Source: three-view drawing plus pictorial views. Frame: mm from the lowest corner of the part. Give positions to 0.01 mm unless a question says otherwise; leave off trailing zeros. Loops run counter-clockwise (first coordinate to the right, second up) from the corner with the lowest first, then second, coordinate; pieces in that order, holes last. Notation, with made-up numbers: (3.5, 64) -> (47.5, 64) arc R25 ccw to (47.5, 81) -> close; hole circle Ø2 at (-1.5, 67.25). An arc over 180 degrees is marked (long way). Answer as a JSON object with one key per item and string values. Group by question number.
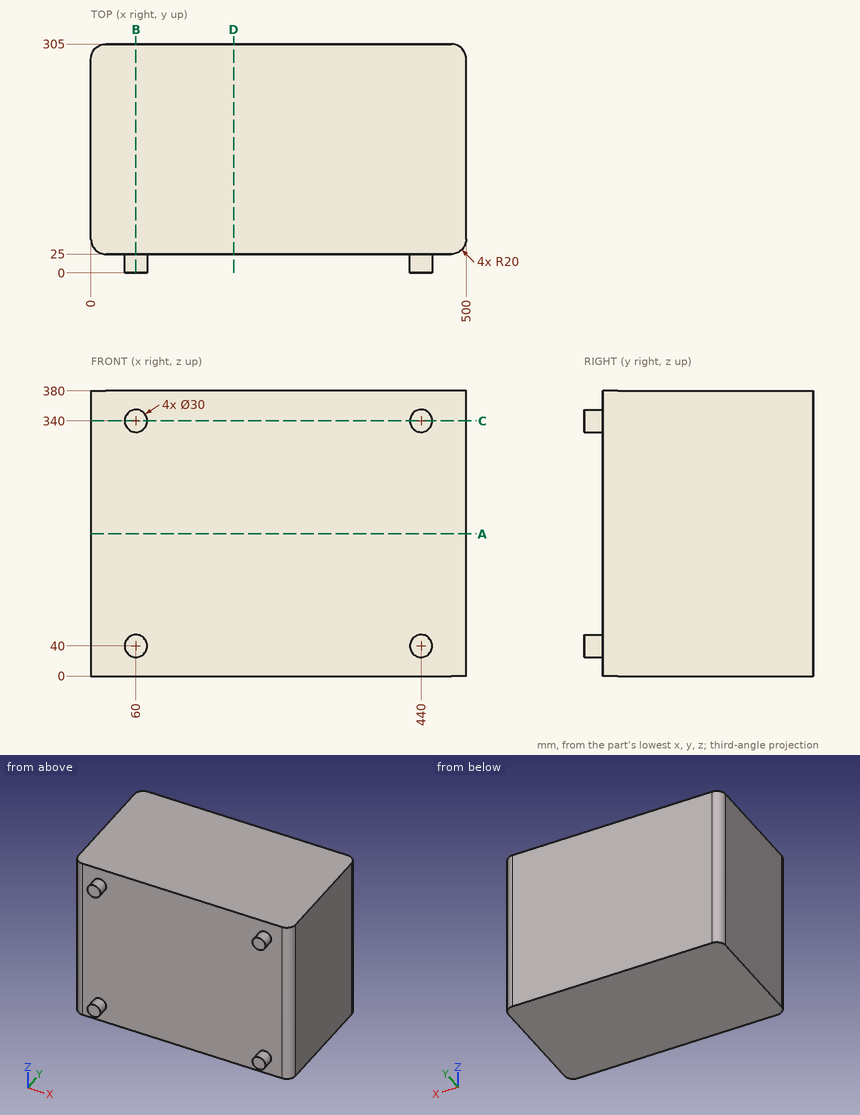
Q1. Section B-B on x = 60. Return the cut outline in (y, z), then the cut area to 3 significant figures.
Q2. Pin query (flat end, axial travel): pin 1 Ø1.5 at (x, y) = (120.5, 48.5) entering from -Z. Return the tip coordinate at first contact, or that it passes through.
Q3. Section A-A on z = 189.5. Return the cut outline in (x, y), then the cut area to 3 significant figures.
Q4. Ray query, probe 1 along Y at (x, z) = (323.5, 36.5). Return the intervals inside material, ascending.
Q5. Section D-D on x = 190. Return the cut outline in (y, z).
Q6. Section C-C on z = 340. Return the cut outline in (x, y).
Numbers:
{
 "1": {"outline": "(0, 25) -> (25, 25) -> (25, 0) -> (305, 0) -> (305, 380) -> (25, 380) -> (25, 355) -> (0, 355) -> (0, 325) -> (25, 325) -> (25, 55) -> (0, 55) -> close", "area": "108,000 mm²"},
 "2": {"pin 1": "stops at z = 0"},
 "3": {"outline": "(0, 45) arc R20 ccw to (20, 25) -> (480, 25) arc R20 ccw to (500, 45) -> (500, 285) arc R20 ccw to (480, 305) -> (20, 305) arc R20 ccw to (0, 285) -> close", "area": "140,000 mm²"},
 "4": {"probe 1": "y = 25 to 305"},
 "5": {"outline": "(25, 0) -> (305, 0) -> (305, 380) -> (25, 380) -> close"},
 "6": {"outline": "(0, 45) arc R20 ccw to (20, 25) -> (45, 25) -> (45, 0) -> (75, 0) -> (75, 25) -> (425, 25) -> (425, 0) -> (455, 0) -> (455, 25) -> (480, 25) arc R20 ccw to (500, 45) -> (500, 285) arc R20 ccw to (480, 305) -> (20, 305) arc R20 ccw to (0, 285) -> close"}
}
